```python
from build123d import *

# Parameters (mm, degrees)
MAIN_DEPTH             = 10
SKETCH4_W              = 20
SKETCH4_H              = 8
INSERT_EXTENSION_DEPTH = 3
SKETCH5_R              = 2.1
INSERT_HOLE_DEPTH      = 5.7


with BuildPart() as part:
    # Sketch2 → Main (new, symmetric)
    with BuildSketch(Plane(origin=(0, 0, 0), x_dir=(0, 0, -1), z_dir=(1, 0, 0))):
        with BuildLine():
            Line((32.5, 0), (40.5, 0))
            add(Edge.make_bspline(
                [(40.5, 0), (40.5, 18), (0, 18)],
                knots=[0, 0, 0, 1.570796327, 1.570796327, 1.570796327], degree=2, weights=[1, 0.707106781, 1]))
            Line((0, 18), (0, 15))
            add(Edge.make_bspline(
                [(32.5, 0), (32.5, 15), (0, 15)],
                knots=[3.141592654, 3.141592654, 3.141592654, 4.71238898, 4.71238898, 4.71238898], degree=2, weights=[1, 0.707106781, 1]))
        make_face()
    main = extrude(amount=MAIN_DEPTH, both=True)

    # Sketch4 → Insert extension (add)
    with BuildSketch(Plane.XZ):
        with Locations((0, -36.5)):
            Rectangle(SKETCH4_W, SKETCH4_H)
    insert_extension = extrude(amount=INSERT_EXTENSION_DEPTH)

    # Sketch5 → Insert hole (cut)
    with BuildSketch(Plane.XZ.offset(3)):
        with Locations(Location((0, -36.5, 0), (0, 0, 270))):
            Circle(SKETCH5_R)
    insert_hole = extrude(amount=-INSERT_HOLE_DEPTH, mode=Mode.SUBTRACT)

    # Mirror1: Main, Insert extension, Insert hole across plane
    add(main.mirror(Plane(origin=(10, 15, 0), x_dir=(1, 0, 0), z_dir=(0, 0, -1))))
    add(insert_extension.mirror(Plane(origin=(10, 15, 0), x_dir=(1, 0, 0), z_dir=(0, 0, -1))))
    add(insert_hole.mirror(Plane(origin=(10, 15, 0), x_dir=(1, 0, 0), z_dir=(0, 0, -1))), mode=Mode.SUBTRACT)


solid = part.part
```
Read the model definition and answer for the solid it produces. Units are mm, in the model's axes. A direction names the side the tool comes from. Coordinates: 2 decimals unless noted, no trailing zeros. Write each loop counter-clockwise with the first axis right and the second up, starting at its lowest first coordinate (ties: lowest second). Pieces come first, ordered by that corner, then holes. Notation, with made-up numbers: (88.25, 4) -> (142.25, 4) arc R38 cw to (142.25, 42) -> close; hole circle Ø7 at (68.25, 28.5). An arc over 180 degrees is marked (long way). Write item = value, one per line.
(1) Section A-A on y = -1 is taken. Write down the section's boundary in (x, z).
From the geometry:
outline = (-10, -40.5) -> (10, -40.5) -> (10, -32.5) -> (-10, -32.5) -> close; (-10, 32.5) -> (10, 32.5) -> (10, 40.5) -> (-10, 40.5) -> close; hole circle Ø4.2 at (0, -36.5); hole circle Ø4.2 at (0, 36.5)
(2) Given pin 1 Ø10 at (x, z) = (7, -20) entering from -Y; pin 2 Ø6 at (x, y) = (2.5, 6) entering from -Z; pin 3 Ø6 at (x, z) = (-1, 13) entering from +Y; pin 4 Ø12 at (y, z) = (0, 22.5) entering from +X, each flat-ended and moving along its own axis, determine where each tip first touches the part or whether it passes through.
From the geometry:
pin_1 = 9.58
pin_2 = -39.93
pin_3 = 17.44
pin_4 = through
(3) For a pull along X with two mould halves and no side action, classify faces 4 (the face through (-2.4, -3, 36.4)), 5 (the face through (10, 15.3, 0.2)), 6 (the face through (0.09, -0.19, -34.4)) as +X half, -X half, draft (parallel to the pull), parting line (faces both ways), or undercut.
From the geometry:
face_4 = draft
face_5 = +X half
face_6 = undercut
(4) Which of the six approach directions +Z, -Z, +X, -X, +Y, -Y give full straight-line access (tool end or side, diameter ignored) to faces 1 (the face through (0, -1, -32.5)), 2 (the face through (-2.4, -3, -36.4)), 3 (the face through (0, 2.7, 36))?
From the geometry:
face_1 = +X, -X, -Y
face_2 = +Z, -Z, +X, -X, -Y
face_3 = -Y
(5) Straight lines are drawn through the part: L1, parallel to Z at x = -0.25, y = 0; L2, parallel to Z at x = 1.75, y = 0; L3, parallel to X at y = 0.5, z = -36.5. For each, find the intervals that lie inside material, in ascending order. Write a range as from..to.
From the geometry:
L1 = -40.5..-38.59, -34.41..-32.5, 32.5..34.41, 38.59..40.5
L2 = -40.5..-37.66, -35.34..-32.5, 32.5..35.34, 37.66..40.5
L3 = -10..-2.1, 2.1..10
